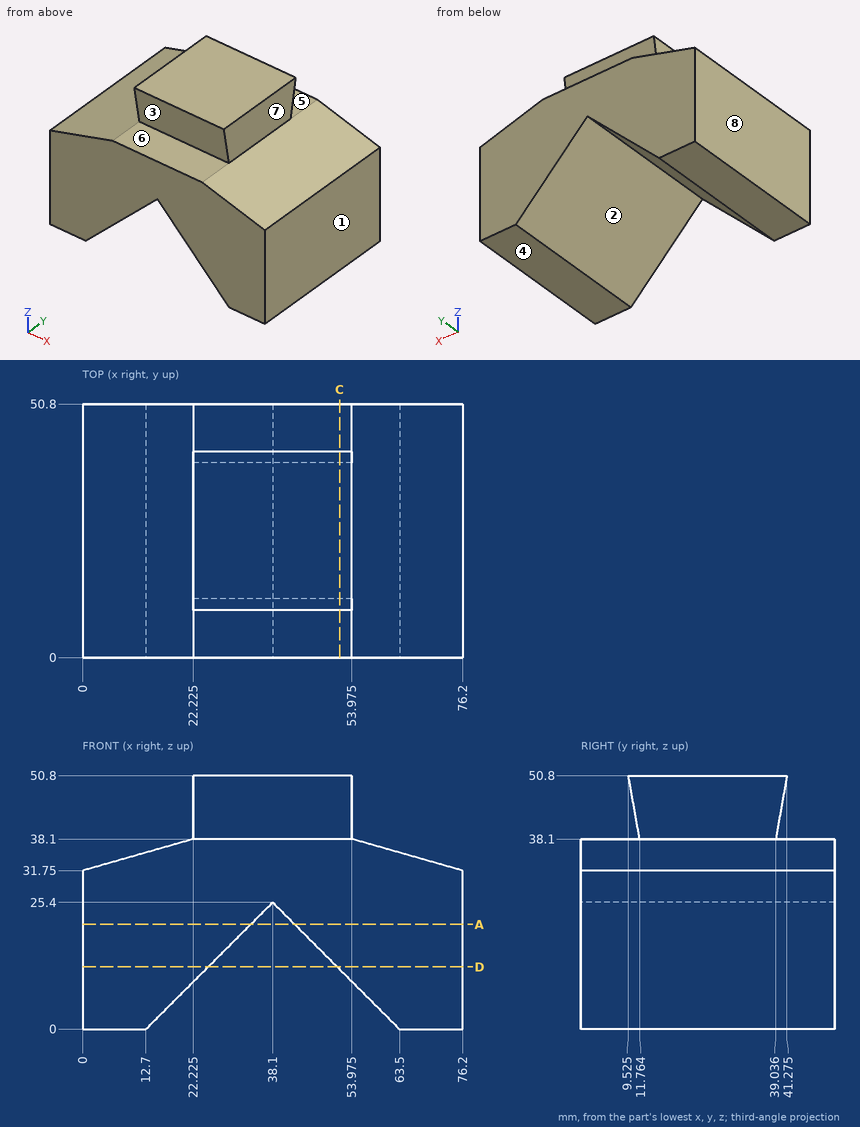
Design review of the part shown in the three views and the two pictorial views. Dimensions are in mm from the part's minimum x, y and z. A direction names the side the tool comes from. Round coordinates to 2 decimals unless told otherwise and drop trailing zeros. Write each loop counter-clockwise with the first axis right and the second up, starting at its lowest first coordinate (ties: lowest second). Pieces come first, ordered by that corner, then holes. Notation, with made-up numbers: (-35.75, 89.5) - (-13.75, 89.5) arc R30 ccw to (-13.75, 128.5) - close; hole circle Ø11 at (-17, 31.5). An arc over 180 degrees is marked (long way). Answer as CSV lines item,"result". Start each with the question number.
(1) Machinability: for the marked faces 4, 5, 6, 7 and 8, which of the approach directions +Z, -Z, +X, -X, +Y, -Y give a long, thin tool a straight path to every point of the face, cutting with its end or side? Answer none if there is none.
(2) For line 1 (X direction, y = 40, z = 46) (1 decimal); line 2 (Z direction, x = 49.5, y = 42); line 3 (X direction, y = 17, z = 22.5), list the stretches that pass through material, from the lowest coordinate up.
(3) For pin 1 (8 mm diameter, centred on x = 15, y = 30.5, fed in from +Z); pin 2 (8 mm diameter, centred on x = 32, z = 36.5, fed in from -Y); pin 3 (6 mm diameter, centred on x = 37.5, y = 9, fed in from -Z); pin 4 (2 mm diameter, centred on x = 22, y = 7.5, fed in from -Z), all flat-tipped, find the tip position at first contact; note any pin that passes through.
(4) Add section D-D, the plane z = 12.5. State the section outline as (x, y) points.
(5) Mouldability with a two-part tool opening along X and no side actions: class the marked faces 1, 2 and 3 as +X half, -X half, draft (parallel to the pull), parting line (faces both ways), or undercut.
(6) Add section A-A, the plane z = 21. State the section outline as (x, y) points, plus the area to 3 significant figures.
(7) Add section C-C, the plane x = 51.5. State the section outline as (y, z) points (1 decimal), plus the area to 3 significant figures.
From the geometry:
1,face 4,"-Z, +X, -X, +Y, -Y"
1,face 5,"+X, -X, +Y"
1,face 6,"+X, -X, -Y"
1,face 7,"+Z, +X, +Y, -Y"
1,face 8,"+Z, -Z, -X, +Y, -Y"
2,line 1,"x = 22.2 to 54"
2,line 2,"z = 14 to 38.1"
2,line 3,"x = 0 to 35.2, 41 to 76.2"
3,pin 1,"stops at z = 37.18"
3,pin 2,"stops at y = 0"
3,pin 3,"stops at z = 21.8"
3,pin 4,"stops at z = 8.3"
4,outline,"(0, 0) - (25.2, 0) - (25.2, 50.8) - (0, 50.8) - close; (51, 0) - (76.2, 0) - (76.2, 50.8) - (51, 50.8) - close"
5,face 1,"+X half"
5,face 2,"undercut"
5,face 3,"draft"
6,outline,"(0, 0) - (33.7, 0) - (33.7, 50.8) - (0, 50.8) - close; (42.5, 0) - (76.2, 0) - (76.2, 50.8) - (42.5, 50.8) - close"
6,area,"3,420 mm²"
7,outline,"(0, 12) - (50.8, 12) - (50.8, 38.1) - (39, 38.1) - (41.3, 50.8) - (9.5, 50.8) - (11.8, 38.1) - (0, 38.1) - close"
7,area,"1,700 mm²"
